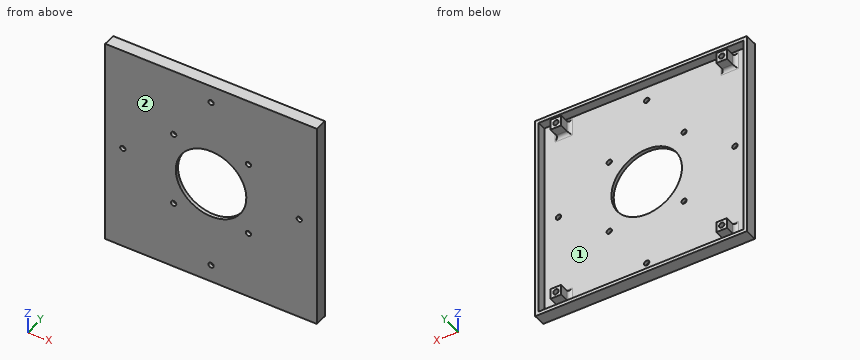
```python
from build123d import *

# Parameters (mm, degrees)
SKETCH1_W           = 116
SKETCH1_H           = 116
SKETCH1_R           = 1.5
SKETCH1_R_2         = 20
BOSS_EXTRUDE1_DEPTH = 2
SKETCH2_W           = 6
SKETCH2_H           = 6
SKETCH2_R           = 1.5
BOSS_EXTRUDE2_DEPTH = 7
SKETCH1_4_W         = 120
SKETCH1_4_H         = 120
SKETCH1_4_W_2       = 116
SKETCH1_4_H_2       = 116
BOSS_EXTRUDE3_DEPTH = 7
SKETCH3_R           = 1.5
CUT_EXTRUDE1_DEPTH  = 86.141059425
FILLET2_R           = 2


with BuildPart() as part:
    # Sketch1 → Boss-Extrude1 (new body)
    with BuildSketch(Plane(origin=(0, 0, 0), x_dir=(1, 0, 0), z_dir=(0, 1, 0))):
        Rectangle(SKETCH1_W, SKETCH1_H)
        with Locations(Location((-21.213203436, -21.213203436, 0), (0, 0, 270))):
            Circle(SKETCH1_R, mode=Mode.SUBTRACT)
        with Locations(Location((21.213203436, 21.213203436, 0), (0, 0, 270))):
            Circle(SKETCH1_R, mode=Mode.SUBTRACT)
        with Locations(Location((0, 0, 0), (0, 0, 270))):
            Circle(SKETCH1_R_2, mode=Mode.SUBTRACT)
        with Locations(Location((-21.213203436, 21.213203436, 0), (0, 0, 270))):
            Circle(SKETCH1_R, mode=Mode.SUBTRACT)
        with Locations(Location((21.213203436, -21.213203436, 0), (0, 0, 270))):
            Circle(SKETCH1_R, mode=Mode.SUBTRACT)
    extrude(amount=BOSS_EXTRUDE1_DEPTH)

    # Sketch2 → Boss-Extrude2 (add)
    # profile 1 of 4: a face of its own
    with BuildSketch(Plane(origin=(0, 2, 0), x_dir=(1, 0, 0), z_dir=(0, 1, 0))):
        with Locations((-47, -52)):
            Rectangle(SKETCH2_W, SKETCH2_H)
        with Locations(Location((-47, -52, 0), (0, 0, 270))):
            Circle(SKETCH2_R, mode=Mode.SUBTRACT)
    # profile 2 of 4: a face of its own
    with BuildSketch(Plane(origin=(0, 2, 0), x_dir=(1, 0, 0), z_dir=(0, 1, 0))):
        with Locations((47, -52)):
            Rectangle(SKETCH2_W, SKETCH2_H)
        with Locations(Location((47, -52, 0), (0, 0, 270))):
            Circle(SKETCH2_R, mode=Mode.SUBTRACT)
    # profile 3 of 4: a face of its own
    with BuildSketch(Plane(origin=(0, 2, 0), x_dir=(1, 0, 0), z_dir=(0, 1, 0))):
        with Locations((47, 52)):
            Rectangle(SKETCH2_W, SKETCH2_H)
        with Locations(Location((47, 52, 0), (0, 0, 270))):
            Circle(SKETCH2_R, mode=Mode.SUBTRACT)
    # profile 4 of 4: a face of its own
    with BuildSketch(Plane(origin=(0, 2, 0), x_dir=(1, 0, 0), z_dir=(0, 1, 0))):
        with Locations((-47, 52)):
            Rectangle(SKETCH2_W, SKETCH2_H)
        with Locations(Location((-47, 52, 0), (0, 0, 270))):
            Circle(SKETCH2_R, mode=Mode.SUBTRACT)
    extrude(amount=BOSS_EXTRUDE2_DEPTH)

    # Sketch1_4 → Boss-Extrude3 (add)
    with BuildSketch(Plane(origin=(0, 0, 0), x_dir=(1, 0, 0), z_dir=(0, 1, 0))):
        Rectangle(SKETCH1_4_W, SKETCH1_4_H)
        Rectangle(SKETCH1_4_W_2, SKETCH1_4_H_2, mode=Mode.SUBTRACT)
    extrude(amount=BOSS_EXTRUDE3_DEPTH)

    # Sketch3 → Cut-Extrude1 (cut, through all)
    with BuildSketch(Plane(origin=(0, 2, 0), x_dir=(1, 0, 0), z_dir=(0, 1, 0))):
        with Locations(Location((50, 0, 0), (0, 0, 270))):
            Circle(SKETCH3_R)
        with Locations(Location((-50, 0, 0), (0, 0, 90))):
            Circle(SKETCH3_R)
        with Locations(Location((0, -50, 0), (0, 0, 270))):
            Circle(SKETCH3_R)
        with Locations(Location((0, 50, 0), (0, 0, 90))):
            Circle(SKETCH3_R)
    extrude(amount=-CUT_EXTRUDE1_DEPTH, mode=Mode.SUBTRACT)

    # Fillet2
    fillet2_edges = [part.edges().sort_by_distance(p)[0] for p in [
        (-47, 2, 49),
        (-50, 2, 52),
        (-47, 2, 55),
        (-44, 2, 52),
        (47, 2, 49),
        (44, 2, 52),
        (50, 2, 52),
        (47, 2, 55),
        (50, 2, -52),
        (47, 2, -55),
        (47, 2, -49),
        (44, 2, -52),
        (-44, 2, -52),
        (-50, 2, -52),
        (-47, 2, -55),
        (-47, 2, -49),
    ]]
    fillet(fillet2_edges, radius=FILLET2_R)


solid = part.part
```
Could you check a few things on this model? Use its own coordinates, in mm. Face numbers are marked on the shaded views. Give positions to 0.01 mm unless a question says otherwise; leave off trailing zeros. Loops run counter-clockwise (first coordinate to the right, second up) from the corner with the lowest first, then second, coordinate; pieces in that order, holes last. Notation, with made-up numbers: (-19, 20) -> (11, 20) arc R17 ccw to (11, 26) -> close; hole circle Ø11 at (77, 8). An arc over 180 degrees is marked (long way). Put each result on its own line as item: value.
(1) Imagine slicing it at B-B on x = 0. Write out the boundary of the cut face in (y, z).
Computed:
outline: (0, -60) -> (7, -60) -> (7, -58) -> (2, -58) -> (2, -51.5) -> (0, -51.5) -> close; (0, -48.5) -> (2, -48.5) -> (2, -20) -> (0, -20) -> close; (0, 20) -> (2, 20) -> (2, 48.5) -> (0, 48.5) -> close; (0, 51.5) -> (2, 51.5) -> (2, 58) -> (7, 58) -> (7, 60) -> (0, 60) -> close
(2) Imagine slicing it at C-C on z = -29. Write out the boundary of the cut face in (x, y), plus the area to 3 significant figures.
Computed:
outline: (-60, 0) -> (60, 0) -> (60, 7) -> (58, 7) -> (58, 2) -> (-58, 2) -> (-58, 7) -> (-60, 7) -> close
area: 260 mm^2
(3) Imagine slicing it at D-D on x = 47. Write out the boundary of the cut face in (y, z).
Computed:
outline: (0, -60) -> (7, -60) -> (7, -58) -> (2, -58) -> (2, -57) arc R2 cw to (4, -55) -> (9, -55) -> (9, -53.5) -> (2, -53.5) -> (2, -50.5) -> (9, -50.5) -> (9, -49) -> (4, -49) arc R2 cw to (2, -47) -> (2, 47) arc R2 cw to (4, 49) -> (9, 49) -> (9, 50.5) -> (2, 50.5) -> (2, 53.5) -> (9, 53.5) -> (9, 55) -> (4, 55) arc R2 cw to (2, 57) -> (2, 58) -> (7, 58) -> (7, 60) -> (0, 60) -> close
(4) Please list where these lines run through material, in increasing order: probe 1 along X at (y, z) = (1.45, 0); probe 2 along Z at (x, y) = (-44.5, 4.25); probe 3 along Z at (x, y) = (-37, 6.75). Write a range as [from, to].
Computed:
probe 1: [-60, -51.5], [-48.5, -20], [20, 48.5], [51.5, 60]
probe 2: [-60, -58], [-55, -49], [49, 55], [58, 60]
probe 3: [-60, -58], [58, 60]
(5) Imagine slicing it at A-A on z = 0. Write out the boundary of the cut face in (x, y), plus the area to 3 significant figures.
Computed:
outline: (-60, 0) -> (-51.5, 0) -> (-51.5, 2) -> (-58, 2) -> (-58, 7) -> (-60, 7) -> close; (-48.5, 0) -> (-20, 0) -> (-20, 2) -> (-48.5, 2) -> close; (20, 0) -> (48.5, 0) -> (48.5, 2) -> (20, 2) -> close; (51.5, 0) -> (60, 0) -> (60, 7) -> (58, 7) -> (58, 2) -> (51.5, 2) -> close
area: 168 mm^2
(6) Thinking about a two-plate mould opening in X: for the marked faces 1 and 2, which applies, pulls with the +X half, pulls with the -X half, needs draft (parallel to the pull), parting line crosses it, or undercut?
Computed:
face 1: undercut
face 2: needs draft
(7) I'm going to push flat-ended pins straight in: pin 1 Ø1.5 at (x, z) = (47, 51.5) entering from +Y; pin 2 Ø3.5 at (x, z) = (47.5, -52.5) entering from +Y. Where does each tip first touch, or does it pass through?
Computed:
pin 1: y = 2
pin 2: y = 9
